Build history of the part. All positions in model axes, mm. A direction names the side the tool comes from. Round coordinates to 2 decimals unless told otherwise and drop trailing zeros. Write each loop counter-clockwise with the first axis right and the second up, starting at its lowest first coordinate (ties: lowest second). Pieces come first, ordered by that corner, then holes. Notation, with made-up numbers: (20.25, 28) - (69.25, 28) arc R20 ccw to (69.25, 55) - close; hole circle Ø11 at (-26.75, 63.25). An arc over 180 degrees is marked (long way). Write each question's results on one line, items separated by ' | '.
Autodesk Inventor part; units mm, degrees
ref_plane "YZ Plane" through (0, 0, 0) normal (1, 0, 0) x (0, 1, 0)
ref_plane "XZ Plane" through (0, 0, 0) normal (0, 1, 0) x (-1, 0, 0)
ref_plane "XY Plane" through (0, 0, 0) normal (0, 0, 1) x (1, 0, 0)
sketch "Sketch1" plane through (0, 0, 0) normal (0, 0, 1) x (1, 0, 0)
  circle A0 centre (0, 0) radius 4.7625
  dimension "max_head_dia" = 9.525
extrude "Extrusion1" add sketch "Sketch1" along normal blind 6.35
sketch "Sketch2" plane through (0, 0, 0) normal (0, 0, -1) x (-1, 0, 0)
  circle A0 centre (0, 0) radius 4.7625
  circle A1 centre (0, 0) radius 3.175
  dimension "max_body_dia" = 6.35
extrude "Extrusion2" add sketch "Sketch2" along normal blind 19.05 contours A1
sketch "Sketch3" plane through (0, 0, 6.35) normal (0, 0, 1) x (1, 0, 0)
  circle A0 centre (0, 0) radius 4.7625
  line L0 (-2.2794, 1.5378) -> (0.192, 2.7429)
  line L1 (0.192, 2.7429) -> (2.4715, 1.2051)
  line L2 (2.4715, 1.2051) -> (2.2794, -1.5378)
  line L3 (2.2794, -1.5378) -> (-0.192, -2.7429)
  line L4 (-0.192, -2.7429) -> (-2.4715, -1.2051)
  line L5 (-2.4715, -1.2051) -> (-2.2794, 1.5378)
  dimension "hex_socket_size" = 4.7625
extrude "Extrusion3" cut sketch "Sketch3" against normal blind 3.048 contours L0 L1 L2 L3 L4 L5
thread "Thread2"
chamfer "Chamfer1" distance 0.635 angle 45 1 edges at (3.175, 0, -19.05)
fillet "Fillet1" radius 0.127 1 edges at (-4.7625, 0, 0)
fillet "Fillet2" radius 0.127 1 edges at (-4.7625, 0, 6.35)
fillet "Fillet3" radius 0.127 6 edges at (-1.3318, -1.974, 6.35) (-2.3754, 0.1663, 6.35) (-1.0437, 2.1403, 6.35) (1.3318, 1.974, 6.35) (2.3754, -0.1663, 6.35) (1.0437, -2.1403, 6.35)
properties part number "4_40_hex_cap_screw"
(1) Drill centre lines: probe 1 along Z at (x, y) = (2.25, -2.5); probe 2 along Z at (x, y) = (2, 0.25); probe 3 along X at (y, z) = (2, -14.75). Where is each one in solid material? Low to high. Write a range as [from, to].
Worked answers:
probe 1: z = [0, 6.35] | probe 2: z = [-19.05, 3.3] | probe 3: x = [-2.47, 2.47]
(2) Two-plate mould, pull along X, no slides. Class faces 4 (the flat face through (0, 0, -19.05)), 5 (the cylindrical face through (0.69, 3.1, -9.08)), 6 (the flat face through (1.061, -2.132, 4.783)), 7 (the flat face through (-1.061, 2.132, 4.783)): released by +X, released by -X, zero draft, split by the parting line, or undercut.
Worked answers:
face 4: zero draft | face 5: split by the parting line | face 6: undercut | face 7: undercut
(3) Slice it at A-A, the plane z = -15. Write the cut outline in (x, y) (3 decimals).
Worked answers:
outline: circle Ø6.35 at (0, 0)
(4) Tool access for faces 1 (the flat face through (2, -3, 0)), 2 (the cylindrical face through (-3.78, 2.9, 3.13)), 3 (the flat face through (-2.377, 0.147, 4.783)): list every direction of +Z, -Z, +X, -X, +Y, -Y with a clear straight run to the whole face (end or side of a thin tool).
Worked answers:
face 1: -Z | face 2: +Z, -Z | face 3: +Z
(5) Flat gauge pins, fed straight in: pin 1 Ø5 at (y, z) = (-3, -8.5) entering from +X; pin 2 Ø1.5 at (x, z) = (0.5, -7.5) entering from -Y (3 decimals). Where does each tip first touch, or does it go through?
Worked answers:
pin 1: stops at x = 3.14 | pin 2: stops at y = -3.175
